Read the model definition and answer for the solid it produces. Units are mm, in the model's axes. A direction names the side the tool comes from. Coordinates: 2 decimals unless noted, no trailing zeros. Write each loop counter-clockwise with the first axis right and the second up, starting at its lowest first coordinate (ties: lowest second). Pieces come first, ordered by that corner, then holes. Notation, with made-up numbers: (73, 65.5) -> (103, 65.5) arc R15 cw to (103, 84.5) -> close; hole circle Ø4 at (27, 65.25). An arc over 180 degrees is marked (long way). Return JSON: item names as keys, results as strings.
from build123d import *

# Parameters (mm, degrees)
SKETCH_1_R          = 1.45
EXTRUDE_1_DEPTH     = 3
CUT_EXTRUDE_1_DEPTH = 3
FILLET_1_R          = 3
FILLET_2_R          = 4


with BuildPart() as part:
    # 草图1 → 凸台-拉伸1 (new body)
    with BuildSketch(Plane.XY):
        Polygon((-24.5, -6), (25, -6), (25, 4), (6, 39), (-6, 39), (-24.5, 4), align=None)
        with Locations((-20, 0)):
            Circle(SKETCH_1_R, mode=Mode.SUBTRACT)
        with Locations((20, 0)):
            Circle(SKETCH_1_R, mode=Mode.SUBTRACT)
        with Locations((0, 35)):
            Circle(SKETCH_1_R, mode=Mode.SUBTRACT)
        with Locations((0, 15)):
            Circle(SKETCH_1_R, mode=Mode.SUBTRACT)
        Circle(SKETCH_1_R, mode=Mode.SUBTRACT)
        with BuildLine():
            Line((-3, 30.192295018), (-3, 3))
            Line((-3, 3), (-21.635270706, 3))
            Line((-21.635270706, 3), (-6.768189881, 31.126909669))
            ThreePointArc((-6.768189881, 31.126909669), (-4.518533366, 32.133477616), (-3, 30.192295018))
        make_face(mode=Mode.SUBTRACT)
        with BuildLine():
            Line((21.635270706, 3), (6.768189881, 31.126909669))
            ThreePointArc((6.768189881, 31.126909669), (4.518533366, 32.133477616), (3, 30.192295018))
            Line((3, 30.192295018), (3, 3))
            Line((3, 3), (21.635270706, 3))
        make_face(mode=Mode.SUBTRACT)
    extrude(amount=EXTRUDE_1_DEPTH)

    # 草图3 → 切除-拉伸1 (cut)
    with BuildSketch(Plane.XY.offset(3)):
        Polygon((-17, -6), (-15, -1), (-6, -1), (-3, -6), align=None)
        Polygon((3, -6), (17, -6), (15, -1), (6, -1), align=None)
    extrude(amount=-CUT_EXTRUDE_1_DEPTH, mode=Mode.SUBTRACT)

    # 圆角1
    fillet_1_edges = [part.edges().sort_by_distance(p)[0] for p in [
        (-24.5, 4, 1.5),
        (-6, 39, 1.5),
        (6, 39, 1.5),
        (25, 4, 1.5),
        (25, -6, 1.5),
        (-24.5, -6, 1.5),
        (-3, -6, 1.5),
        (-17, -6, 1.5),
        (-15, -1, 1.5),
        (-6, -1, 1.5),
        (3, -6, 1.5),
        (6, -1, 1.5),
        (15, -1, 1.5),
        (17, -6, 1.5),
    ]]
    fillet(fillet_1_edges, radius=FILLET_1_R)

    # 圆角2
    fillet_2_edges = [part.edges().sort_by_distance(p)[0] for p in [
        (-21.635270706, 3, 1.5),
        (-3, 3, 1.5),
        (3, 3, 1.5),
        (21.635270706, 3, 1.5),
    ]]
    fillet(fillet_2_edges, radius=FILLET_2_R)


solid = part.part
1. The part is cut by section C-C (x = -10.5). Determine the outline of the cut face in (y, z), then the cut area to 3 significant figures.
Taken from the geometry:
{"outline": "(-1, 0) -> (3, 0) -> (3, 3) -> (-1, 3) -> close; (24.07, 0) -> (30.49, 0) -> (30.49, 3) -> (24.07, 3) -> close", "area": "31.3 mm2"}
2. The part is cut by section A-A (y = 0). Determine the outline of the cut face in (x, z).
Taken from the geometry:
{"outline": "(-24.5, 0) -> (-21.45, 0) -> (-21.45, 3) -> (-24.5, 3) -> close; (-18.55, 0) -> (-1.45, 0) -> (-1.45, 3) -> (-18.55, 3) -> close; (1.45, 0) -> (18.55, 0) -> (18.55, 3) -> (1.45, 3) -> close; (21.45, 0) -> (25, 0) -> (25, 3) -> (21.45, 3) -> close"}
3. The part is cut by section D-D (y = 23). Determine the outline of the cut face in (x, z).
Taken from the geometry:
{"outline": "(-14.46, 0) -> (-11.06, 0) -> (-11.06, 3) -> (-14.46, 3) -> close; (-3, 0) -> (3, 0) -> (3, 3) -> (-3, 3) -> close; (11.06, 0) -> (14.69, 0) -> (14.69, 3) -> (11.06, 3) -> close"}
4. A tool of negligible diameter and unlimited length cuts with its end or side. For faces 4 (the face through (2, 12, 0)), 5 (the face through (-3, 19, 1)), 6 (the face through (-2.8, -5.6, 1.5)), from which of +Z, -Z, +X, -X, +Y, -Y can it reach the whole face along a straight path? Write none if from no direction.
Taken from the geometry:
{"face 4": "-Z, +X, -X, +Y, -Y", "face 5": "+Z, -Z", "face 6": "+Z, -Z, -Y"}
5. The part is cut by section B-B (x = 0). Determine the outline of the cut face in (y, z).
Taken from the geometry:
{"outline": "(-6, 0) -> (-1.45, 0) -> (-1.45, 3) -> (-6, 3) -> close; (1.45, 0) -> (13.55, 0) -> (13.55, 3) -> (1.45, 3) -> close; (16.45, 0) -> (33.55, 0) -> (33.55, 3) -> (16.45, 3) -> close; (36.45, 0) -> (39, 0) -> (39, 3) -> (36.45, 3) -> close"}
6. Consider L1, parallel to Y at x = 0, z = 1.9; L2, parallel to X at y = 4.5, z = 2.4; L3, parallel to Y at x = -1, z = 0.85. Determine where each line is inside the solid, lowest interval first.
Taken from the geometry:
{"L1": "y = -6 to -1.45, 1.45 to 13.55, 16.45 to 33.55, 36.45 to 39", "L2": "x = -24.23 to -18.12, -3.88 to 3.88, 18.12 to 24.72", "L3": "y = -6 to -1.05, 1.05 to 13.95, 16.05 to 33.95, 36.05 to 39"}
7. For a pull along Y with two mould halves and no side action, classify faces 1 (the face through (2, 12, 3)), 2 (the face through (-23.6, -5.14, 1.52)), 3 (the face through (0.669, 33.714, 1.479)) as +Y half, -Y half, draft (parallel to the pull), parting line (faces both ways), or undercut.
Taken from the geometry:
{"face 1": "draft", "face 2": "-Y half", "face 3": "undercut"}
8. Flat-ended cylindrical pins translate along their axes: pin 1 Ø1.5 at (x, z) = (10.5, 1) entering from +Y; pin 2 Ø1.5 at (x, z) = (11, 1) entering from -Y; pin 3 Ø1.5 at (y, z) = (24, 1.5) entering from -X (3 decimals). Find the tip coordinate at first contact, or state that the pin passes through.
Taken from the geometry:
{"pin 1": "stops at y = 32.09", "pin 2": "stops at y = -1", "pin 3": "stops at x = -14.325"}
